from build123d import *

# Parameters (mm, degrees)
SKETCH019_R             = 10
PAD019_DEPTH            = 17
SKETCH020_R             = 9
POCKET_DEPTH            = 4.2
SKETCH021_R             = 3
POCKET001_DEPTH         = 11.8
BODY009_PLACEMENT_ANGLE = 180


with BuildPart() as part:
    # Sketch019 → Pad019 (new body)
    with BuildSketch(Plane.XY):
        Circle(SKETCH019_R)
    extrude(amount=PAD019_DEPTH)

    # Sketch020 (on Face2 of Pad019) → Pocket (cut)
    with BuildSketch(Plane(origin=(0, 0, 0), x_dir=(1, 0, 0), z_dir=(0, 0, -1))):
        Circle(SKETCH020_R)
    extrude(amount=-POCKET_DEPTH, mode=Mode.SUBTRACT)

    # Sketch021 (on Face5 of Pocket) → Pocket001 (cut)
    with BuildSketch(Plane(origin=(0, 0, 4.2), x_dir=(1, 0, 0), z_dir=(0, 0, -1))):
        Circle(SKETCH021_R)
    extrude(amount=-POCKET001_DEPTH, mode=Mode.SUBTRACT)


with BuildPart() as part_1:
    # Body009 placement: moved
    add(part.part.moved(Location((-5, 7, -16.4))).rotate(Axis((-5, 7, -16.4), (1, 0, 0)), BODY009_PLACEMENT_ANGLE))


solid = part_1.part
Work out the finished part from the listing and answer in its coordinate system (mm). A direction names the side the tool comes from. Round coordinates to 2 decimals unless told otherwise and drop trailing zeros. Write each loop counter-clockwise with the first axis right and the second up, starting at its lowest first coordinate (ties: lowest second). Pieces come first, ordered by that corner, then holes. Notation, with made-up numbers: M 76,-10.75 L 125,-10.75 A18 cw 125,-4.75 Z; hole C 74,83 d7. An arc over 180 degrees is marked long. Use a Markdown table: item, result.
1) Determine the mould class of faces 3 (the face through (-15, 7, -25)), 4 (the face through (-14, 5, -16.4)), 5 (the face through (-5, 7, -32.4)) for opening direction Y: pulls with the +Y half, pulls with the -Y half, needs draft (parallel to the pull), parting line crosses it, or undercut.
Taken from the geometry:
| item | result |
|---|---|
| face 3 | parting line crosses it |
| face 4 | needs draft |
| face 5 | undercut |
2) Flat-ended cylindrical pins translate along their axes: pin 1 (9 mm diameter, centred on x = -3, y = 7.5, fed in from +Z); pin 2 (1.5 mm diameter, centred on x = -7.5, z = -31.5, fed in from +Y); pin 3 (4 mm diameter, centred on x = 0.5, z = -22.5, fed in from -Y). Find the tip coordinate at first contact, or state that the pin passes through.
Taken from the geometry:
| item | result |
|---|---|
| pin 1 | stops at z = -20.6 |
| pin 2 | stops at y = 16.85 |
| pin 3 | stops at y = -2.37 |
3) The part is cut by section C-C on x = -10. Give the vertices of the cut face in (y, z).
Taken from the geometry:
| item | result |
|---|---|
| outline | M -1.66,-33.4 L 15.66,-33.4 L 15.66,-16.4 L 14.48,-16.4 L 14.48,-20.6 L -0.48,-20.6 L -0.48,-16.4 L -1.66,-16.4 Z |
4) The part is cut by section B-B on z = -18.5. Give the vertices of the cut face in (x, y).
Taken from the geometry:
| item | result |
|---|---|
| outline | C -5,7 d20; hole C -5,7 d18 |
5) The part is cut by section D-D on y = -0.75. Give the vertices of the cut face in (x, z).
Taken from the geometry:
| item | result |
|---|---|
| outline | M -11.32,-33.4 L 1.32,-33.4 L 1.32,-16.4 L -0.42,-16.4 L -0.42,-20.6 L -9.58,-20.6 L -9.58,-16.4 L -11.32,-16.4 Z |
6) The part is cut by section A-A on y = 7. Give the vertices of the cut face in (x, z).
Taken from the geometry:
| item | result |
|---|---|
| outline | M -15,-33.4 L 5,-33.4 L 5,-16.4 L 4,-16.4 L 4,-20.6 L -2,-20.6 L -2,-32.4 L -8,-32.4 L -8,-20.6 L -14,-20.6 L -14,-16.4 L -15,-16.4 Z |
7) Which of the six approach directions +Z, -Z, +X, -X, +Y, -Y give full straight-line access (tool end or side, diameter ignored) to faces 1 (the face through (-5, 7, -33.4)), 2 (the face through (-5.65, 4.07, -26.42))?
Taken from the geometry:
| item | result |
|---|---|
| face 1 | -Z, +X, -X, +Y, -Y |
| face 2 | +Z |
8) Consider line 1 (Y direction, x = -5, z = -25); line 2 (Y direction, x = -5, z = -18.05); line 3 (Z direction, x = -11, y = 10.75). Determine where each line is inside the solid, lowest interval first. Write a range as [from, to].
Taken from the geometry:
| item | result |
|---|---|
| line 1 | y = [-3, 4], [10, 17] |
| line 2 | y = [-3, -2], [16, 17] |
| line 3 | z = [-33.4, -20.6] |
